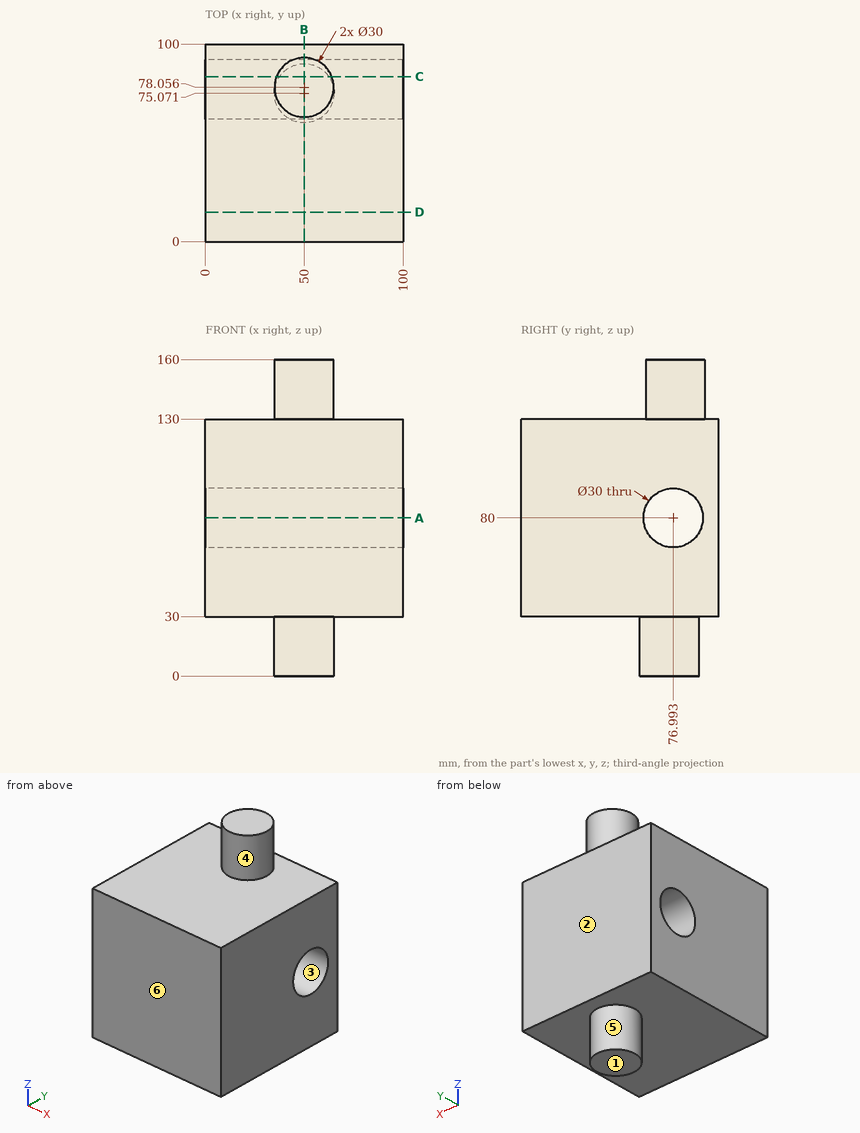
Geometry: see drawing. Coordinates: mm, zero at the bounding-box minimum. A direction names the side the tool comes from. Round coordinates to 2 decimals unless told otherwise and drop trailing zeros. Write each loop counter-clockwise with the first axis right and the second up, starting at its lowest first coordinate (ties: lowest second). Pieces come first, ordered by that corner, then holes.
1) Cut plane A-A (z = 80). Return the cut outline in (x, y), then the cut area to 3 significant figures.
2) Cut plane B-B (x = 50). Return the cut outline in (y, z).
3) Contact query for flat-ended pins moving along their axis: P1, Ø24, axis at y = 76.99, z = 80, coming from the -X side; P2, Ø8, axis at y = 56, z = 78.5, coming from the -X side; P3, Ø2, axis at y = 65.5, z = 137.5, coming from the +X side (1 decimal); P4, Ø5, axis at x = 89, y = 39, coming from the -Z side. Output: stop coordinate, or through.
4) Ray query, L1, parallel to Z at x = 14, y = 11.5; L2, parallel to Z at x = 52.5, y = 78.5 (1 decimal); L3, parallel to Y at x = 66, z = 86 (1 decimal). Return the intervals inside material, ascending.
5) Cut plane C-C (y = 83.5). Return the cut outline in (x, z) (1 decimal).
6) Draft query along Z for the marked faces 1, 2 and 3. Return one class per face: pulls with the +Z half, pulls with the -Z half, needs draft (parallel to the pull), parting line crosses it, or undercut.
7) Reachability of the marked faces 4, 5 and 6 from +Z, -Z, +X, -X, +Y, -Y: full face, straight path, thin tool, end or side. Return the list, or none.
8) Cut plane D-D (y = 15). Return the cut outline in (x, z).
Geometry says:
1. outline: (0, 0) - (100, 0) - (100, 61.99) - (0, 61.99) - close; (0, 91.99) - (100, 91.99) - (100, 100) - (0, 100) - close
1. area: 7,000 mm2
2. outline: (0, 30) - (60.07, 30) - (60.07, 0) - (90.07, 0) - (90.07, 30) - (100, 30) - (100, 130) - (93.06, 130) - (93.06, 160) - (63.06, 160) - (63.06, 130) - (0, 130) - close; hole circle Ø30 at (76.99, 80)
3. P1: passes through
3. P2: stops at x = 0
3. P3: stops at x = 59.6
3. P4: stops at z = 30
4. L1: z = 30 to 130
4. L2: z = 0 to 65.1, 94.9 to 160
4. L3: y = 0 to 63.2, 90.7 to 100
5. outline: (0, 30) - (37.6, 30) - (37.6, 0) - (62.4, 0) - (62.4, 30) - (100, 30) - (100, 66.5) - (0, 66.5) - close; (0, 93.5) - (100, 93.5) - (100, 130) - (64, 130) - (64, 160) - (36, 160) - (36, 130) - (0, 130) - close
6. face 1: pulls with the -Z half
6. face 2: needs draft
6. face 3: undercut
7. face 4: +Z
7. face 5: -Z
7. face 6: +Z, -Z, +X, -X, -Y
8. outline: (0, 30) - (100, 30) - (100, 130) - (0, 130) - close
